```python
from build123d import *
from OCP.BRepFilletAPI import BRepFilletAPI_MakeFillet

# Parameters (mm, degrees)
BOSS_EXTRUDE1_DEPTH = 12.7
BOSS_EXTRUDE2_START = 10.16
BOSS_EXTRUDE2_DEPTH = 10.16
CUT_EXTRUDE1_REACH  = 103.575
SKETCH5_R           = 1.651
CUT_EXTRUDE2_DEPTH  = 104.355902105
FILLET1_R1          = 0.508
FILLET1_R2          = 1.27


with BuildPart() as part:
    # Sketch1 → Boss-Extrude1 (new body)
    with BuildSketch(Plane(origin=(0, 0, 0), x_dir=(1, 0, 0), z_dir=(0, 1, 0))):
        with BuildLine():
            Line((2.54, -3.81), (83.46, -3.81))
            ThreePointArc((83.46, -3.81), (87.950128061, -1.950128061), (89.81, 2.54))
            Line((89.81, 2.54), (89.81, 35.56))
            ThreePointArc((89.81, 35.56), (87.950128061, 40.050128061), (83.46, 41.91))
            Line((83.46, 41.91), (2.54, 41.91))
            ThreePointArc((2.54, 41.91), (-1.950128061, 40.050128061), (-3.81, 35.56))
            Line((-3.81, 35.56), (-3.81, 2.54))
            ThreePointArc((-3.81, 2.54), (-1.950128061, -1.950128061), (2.54, -3.81))
        make_face()
        with BuildLine():
            Line((2.54, 0), (83.46, 0))
            ThreePointArc((83.46, 0), (85.256051224, 0.743948776), (86, 2.54))
            Line((86, 2.54), (86, 35.56))
            ThreePointArc((86, 35.56), (85.256051224, 37.356051224), (83.46, 38.1))
            Line((83.46, 38.1), (2.54, 38.1))
            ThreePointArc((2.54, 38.1), (0.743948776, 37.356051224), (0, 35.56))
            Line((0, 35.56), (0, 2.54))
            ThreePointArc((0, 2.54), (0.743948776, 0.743948776), (2.54, 0))
        make_face(mode=Mode.SUBTRACT)
    extrude(amount=-BOSS_EXTRUDE1_DEPTH)

    # Sketch3 → Boss-Extrude2 (add)
    with BuildSketch(Plane(origin=(0, 0, 0), x_dir=(1, 0, 0), z_dir=(0, 1, 0)).offset(BOSS_EXTRUDE2_START)):
        with BuildLine():
            Line((83.46, 41.91), (2.54, 41.91))
            ThreePointArc((2.54, 41.91), (-1.950128061, 40.050128061), (-3.81, 35.56))
            Line((-3.81, 35.56), (-3.81, 2.54))
            ThreePointArc((-3.81, 2.54), (-1.950128061, -1.950128061), (2.54, -3.81))
            Line((2.54, -3.81), (83.46, -3.81))
            ThreePointArc((83.46, -3.81), (87.950128061, -1.950128061), (89.81, 2.54))
            Line((89.81, 2.54), (89.81, 35.56))
            ThreePointArc((89.81, 35.56), (87.950128061, 40.050128061), (83.46, 41.91))
        make_face()
    extrude(amount=-BOSS_EXTRUDE2_DEPTH)

    # Sketch4 → Cut-Extrude1 (cut, up to next)
    with BuildSketch(Plane.XY.offset(3.81), mode=Mode.PRIVATE) as cut_extrude1_sk1:
        Polygon((73.3, 10.16), (73.3, 8.255), (80.92, 8.255), (80.92, 3.81), (5.08, 3.81), (5.08, 8.255), (12.7, 8.255), (12.7, 10.16), align=None)
    cut_extrude1_tool1 = extrude(cut_extrude1_sk1.sketch, amount=-CUT_EXTRUDE1_REACH, mode=Mode.PRIVATE) & part.part
    add(cut_extrude1_tool1.solids().sort_by_distance((43, 6.842422, 3.81))[0], mode=Mode.SUBTRACT)

    # Sketch5 → Cut-Extrude2 (cut, through all)
    with BuildSketch(Plane(origin=(89.81, 0, 0), x_dir=(0, 0, -1), z_dir=(1, 0, 0))):
        with Locations((19.05, 5.8325)):
            Circle(SKETCH5_R)
    extrude(amount=-CUT_EXTRUDE2_DEPTH, mode=Mode.SUBTRACT)

    # Fillet1: one fillet with a radius per group of edges: ONE call of the kernel's fillet builder (fillet() takes one radius for all edges)
    fillet1_edges_1 = [part.edges().sort_by_distance(p)[0] for p in [
        (12.7, 8.255, -19.05),
        (73.3, 8.255, -19.05),
        (12.7, 10.16, -19.05),
        (73.3, 10.16, -19.05),
        (7.62, 10.16, -41.91),
        (78.38, 10.16, -41.91),
    ]]
    fillet1_edges_2 = [part.edges().sort_by_distance(p)[0] for p in [
        (43, -12.7, 0),
    ]]
    fillet1 = BRepFilletAPI_MakeFillet(part.part.solid().wrapped)
    for e in fillet1_edges_1:
        fillet1.Add(FILLET1_R1, e.wrapped)
    for e in fillet1_edges_2:
        fillet1.Add(FILLET1_R2, e.wrapped)
    add(Compound.cast(fillet1.Shape()), mode=Mode.REPLACE)


solid = part.part
```
Input: part model. Units: mm. Frame: model coordinates. A direction names the side the tool comes from. Round coordinates to 2 decimals unless told otherwise and drop trailing zeros. Loops run counter-clockwise (first coordinate to the right, second up) from the corner with the lowest first, then second, coordinate; pieces in that order, holes last. Notation, with made-up numbers: M 61,14.5 L 116,14.5 A13 ccw 116,26.5 Z; hole C -21.5,83 d7. An arc over 180 degrees is marked long. Answer in a Markdown table with one row per item. Add a question column.
1. Section A-A (y = -10.5). Output: boundary loops of the cut face in (x, z), and give its area (3 significant figures).
2. Section D-D (x = 4). Output: boundary loops of the cut face in (y, z).
3. Mould query, pull axis X, two halves, no side actions, for faces 1 (the face through (88, -1, -40)), 2 (the face through (5.08, 8, -19)), 3 (the face through (4, 10.16, -19)). Classes: released by +X, released by -X, zero draft, split by the parting line, or undercut.
4. Section C-C (x = 19.5). Output: boundary loops of the cut face in (y, z).
5. Set-up query: faces 4 (the face through (81, 10.16, -19)), 5 (the face through (0.724, -5.635, -0.764)), 6 (the face through (9, 8.255, -19)). Return all of +Z, -Z, +X, -X, +Y, -Y with unobstructed straight access to the full face (end or side cutting, diameter ignored); none if empty.
6. Ray query, probe 1 along X at (y, z) = (-7.25, -35.5); probe 2 along X at (y, z) = (8, -17); probe 3 along Z at (x, y) = (47.5, -11.25). Return the intervals inside material, ascending.
7. Contact query for flat-ended pins moving along their axis: pin 1 (3.5 mm diameter, centred on x = 10, z = -10.5, fed in from -Y); pin 2 (13.5 mm diameter, centred on x = 52.5, z = -19.5, fed in from +Y). Output: stop coordinate, or through.
8. Section B-B (z = -19.05). Give the number of separate pieces and of enclosed holes in the cut face, and give its area (3 significant figures).
Values follow:
| question | item | result |
|---|---|---|
| 1 | outline | M -3.81,-35.56 A6.35 ccw 2.54,-41.91 L 83.46,-41.91 A6.35 ccw 89.81,-35.56 L 89.81,-2.54 A6.35 ccw 83.46,3.81 L 2.54,3.81 A6.35 ccw -3.81,-2.54 Z; hole M 0,-35.56 A2.54 ccw 2.54,-38.1 L 83.46,-38.1 A2.54 ccw 86,-35.56 L 86,-2.54 A2.54 ccw 83.46,0 L 2.54,0 A2.54 ccw 0,-2.54 Z |
| 1 | area | 975 mm^2 |
| 2 | outline | M -12.7,-41.91 L 9.65,-41.91 A0.51 ccw 10.16,-41.4 L 10.16,3.3 A0.51 ccw 9.65,3.81 L -12.7,3.81 L -12.7,1.27 A1.27 ccw -11.43,0 L 0,0 L 0,-38.1 L -11.43,-38.1 A1.27 ccw -12.7,-39.37 Z; hole C 5.83,-19.05 d3.3 |
| 3 | face 1 | released by +X |
| 3 | face 2 | undercut |
| 3 | face 3 | zero draft |
| 4 | outline | M -12.7,-41.91 L 3.81,-41.91 L 3.81,3.81 L -12.7,3.81 L -12.7,1.27 A1.27 ccw -11.43,0 L 0,0 L 0,-38.1 L -11.43,-38.1 A1.27 ccw -12.7,-39.37 Z |
| 5 | face 4 | +Z, -Z, +X, -X, +Y |
| 5 | face 5 | -Y |
| 5 | face 6 | +Z, -Z |
| 6 | probe 1 | -3.81 to 0, 86 to 89.81 |
| 6 | probe 2 | -3.81 to 5.08, 80.92 to 89.81 |
| 6 | probe 3 | -41.91 to -38.1, 0 to 3.81 |
| 7 | pin 1 | y = 0 |
| 7 | pin 2 | y = 3.81 |
| 8 | separate pieces | 3 |
| 8 | enclosed holes | 0 |
| 8 | area | 536 mm^2 |
